Check sheet for the modelled part. Datum: model origin and axes. Units: mm. Give positions to 0.01 mm unless a question says otherwise; leave off trailing zeros. Write each loop counter-clockwise with the first axis right and the second up, starting at its lowest first coordinate (ties: lowest second). Pieces come first, ordered by that corner, then holes. Notation, with made-up numbers: M 62,21.5 L 69,21.5 A34 ccw 69,53.5 Z; hole C 1,-25.5 d3. An arc over 180 degrees is marked long. Write item = value, one per line. Start each with the question number.
1) Gauge pin test, flat end, axial feed: pin 1 (4 mm diameter, centred on x = 2, y = 34.5, fed in from +Z). Record the tip position at first contact, or that the pin passes through.
2) Draft check along X on faces 1 (the face through (-13.5, 38, 1)), 2 (the face through (0, 200, 0)), 3 (the face through (0, 42, 2)). Enter one of: pulls with the +X half, pulls with the -X half, needs draft (parallel to the pull), parting line crosses it, or undercut.
3) Sectioned sample at B-B, the plane x = -3.75. Record the cut outline in (y, z), then the cut area to 3 significant figures.
4) Scan lines: L1, parallel to X at y = 71.5, z = 2.75; L2, parallel to Z at x = 1, y = 90.5. Record each from-to range of solid material in increasing order.
5) Sectioned sample at A-A, the plane y = -85. Record the cut outline in (x, z), then the cut area to 3 significant figures.
from build123d import *

# Parameters (mm, degrees)
SCHIZZO1_W                        = 6.5
SCHIZZO1_H                        = 80
ESTRUSIONE_ESTRUSIONE1_DEPTH      = 2
SCHIZZO2_W                        = 3
SCHIZZO2_H                        = 320
ESTRUSIONE_ESTRUSIONE2_DEPTH      = 7
SMUSSO1_SIZE                      = 1
SCHIZZO4_W                        = 3
SCHIZZO4_H                        = 1
TAGLIO_ESTRUSIONE1_DEPTH          = 321.298688727
SMUSSO1_OF_SPECCHIA9_SIZE         = 1
ESTRUSIONE_ESTRUSIONE3_DEPTH      = 122
ESTRUSIONE_ESTRUSIONE3_DEPTH_BACK = 200
SCHIZZO5_W                        = 13
SCHIZZO5_H                        = 2
SCHIZZO6_W                        = 13
SCHIZZO6_H                        = 2
TAGLIO_ESTRUSIONE2_DEPTH          = 2
ESTRUSIONE_ESTRUSIONE4_DEPTH      = 2
ESTRUSIONE_ESTRUSIONE5_DEPTH      = 2


with BuildPart() as part:
    # Schizzo1 → Estrusione-Estrusione1 (new body)
    with BuildSketch(Plane.XY):
        with Locations((3.25, 40)):
            Rectangle(SCHIZZO1_W, SCHIZZO1_H)
    estrusione_estrusione1 = extrude(amount=ESTRUSIONE_ESTRUSIONE1_DEPTH)

    # Schizzo2 → Estrusione-Estrusione2 (add)
    with BuildSketch(Plane(origin=(6.5, 0, 0), x_dir=(0, 0, -1), z_dir=(1, 0, 0))):
        with Locations((-1.5, 40)):
            Rectangle(SCHIZZO2_W, SCHIZZO2_H)
    estrusione_estrusione2 = extrude(amount=ESTRUSIONE_ESTRUSIONE2_DEPTH)

    # Smusso1
    smusso1_edges = [part.edges().sort_by_distance(p)[0] for p in [
        (6.5, 200, 1.5),
        (6.5, -120, 1.5),
        (13.5, 200, 1.5),
        (13.5, -120, 1.5),
    ]]
    chamfer(smusso1_edges, length=SMUSSO1_SIZE)

    # Schizzo4 → Taglio-Estrusione1 (cut, through all)
    with BuildSketch(Plane.XZ.offset(120)):
        with Locations((10, 2.5)):
            Rectangle(SCHIZZO4_W, SCHIZZO4_H)
    taglio_estrusione1 = extrude(amount=-TAGLIO_ESTRUSIONE1_DEPTH, mode=Mode.SUBTRACT)

    # Specchia9: Estrusione-Estrusione1, Estrusione-Estrusione2, Taglio-Estrusione1 across plane
    add(estrusione_estrusione1.mirror(Plane.ZY))
    add(estrusione_estrusione2.mirror(Plane.ZY))
    add(taglio_estrusione1.mirror(Plane.ZY), mode=Mode.SUBTRACT)

    # Smusso1 of Specchia9
    smusso1_of_specchia9_edges = [part.edges().sort_by_distance(p)[0] for p in [
        (-6.5, 200, 1.5),
        (-6.5, -120, 1.5),
        (-13.5, 200, 1.5),
        (-13.5, -120, 1.5),
    ]]
    chamfer(smusso1_of_specchia9_edges, length=SMUSSO1_OF_SPECCHIA9_SIZE)

    # Schizzo5 → Estrusione-Estrusione3 (add, two sides: drawn at the far end of the back side and taken through both)
    with BuildSketch(Plane.XZ.offset(-ESTRUSIONE_ESTRUSIONE3_DEPTH_BACK)):
        with Locations((0, 1)):
            Rectangle(SCHIZZO5_W, SCHIZZO5_H)
    extrude(amount=ESTRUSIONE_ESTRUSIONE3_DEPTH + ESTRUSIONE_ESTRUSIONE3_DEPTH_BACK)

    # Schizzo6 → Taglio-Estrusione2 (cut)
    with BuildSketch(Plane.XZ.offset(122)):
        with Locations((0, 1)):
            Rectangle(SCHIZZO6_W, SCHIZZO6_H)
    extrude(amount=-TAGLIO_ESTRUSIONE2_DEPTH, mode=Mode.SUBTRACT)

    # Schizzo7 → Estrusione-Estrusione4 (add)
    with BuildSketch(Plane(origin=(0, 0, 0), x_dir=(-1, 0, 0), z_dir=(0, 0, -1))):
        Polygon((-7.5, 200), (-6.5, 200), (-6.5, 199), align=None)
        Polygon((6.5, 200), (6.5, 199), (7.5, 200), align=None)
        Polygon((-7.5, -120), (-6.5, -120), (-6.5, -119), align=None)
        Polygon((6.5, -119), (6.5, -120), (7.5, -120), align=None)
    extrude(amount=-ESTRUSIONE_ESTRUSIONE4_DEPTH)

    # Schizzo8 → Estrusione-Estrusione5 (add)
    with BuildSketch(Plane(origin=(0, 0, 0), x_dir=(-1, 0, 0), z_dir=(0, 0, -1))):
        Polygon((-13.5, -119), (-12.5, -120), (12.5, -120), (13.5, -119), (13.5, 199), (12.5, 200), (-12.5, 200), (-13.5, 199), align=None)
    extrude(amount=ESTRUSIONE_ESTRUSIONE5_DEPTH)


solid = part.part
Data:
q1.pin_1 = 2
q2.face_1 = pulls with the -X half
q2.face_2 = needs draft
q2.face_3 = undercut
q3.outline = M -120,-2 L 200,-2 L 200,2 L -120,2 Z
q3.area = 1,280 mm2
q4.L1 = -13.5 to -11.5, -8.5 to -6.5, 6.5 to 8.5, 11.5 to 13.5
q4.L2 = -2 to 2
q5.outline = M -13.5,-2 L 13.5,-2 L 13.5,3 L 11.5,3 L 11.5,2 L 8.5,2 L 8.5,3 L 6.5,3 L 6.5,2 L -6.5,2 L -6.5,3 L -8.5,3 L -8.5,2 L -11.5,2 L -11.5,3 L -13.5,3 Z
q5.area = 116 mm2
